The model under review builds one solid part; all positions refer to its coordinate system, in mm. Face numbers are marked on the shaded views. A direction names the side the tool comes from. Coordinates: 2 decimals unless noted, no trailing zeros. Loops run counter-clockwise (first coordinate to the right, second up) from the corner with the lowest first, then second, coordinate; pieces in that order, holes last. Notation, with made-up numbers: (51, 58.25) - (105, 58.25) arc R15 cw to (105, 76.25) - close; hole circle Ø10 at (78.25, -22). An arc over 180 degrees is marked (long way). Answer in a Markdown table with one row per item. Add a question column.
(1) Mouldability with a two-part tool opening along X and no side actions: class the marked faces 1, 2 and 3 as +X half, -X half, draft (parallel to the pull), parting line (faces both ways), or undercut.
(2) We need section D-D on y = -4. Write out the cut boundary in (x, z) (3 decimals).
(3) We need section A-A on z = 0. Write out the cut boundary in (x, y) (3 decimals), plus the area to 3 significant figures.
(4) For P1, Ø8, axis at x = 14, z = -18, coming from the -Y side; P2, Ø8, axis at y = -17, z = 4, coming from the +X side; P3, Ø2, axis at y = -5, z = -3.5, coming from the +X side, all flat-tipped, find the tip position at first contact; note any pin that passes through.
(5) We need section C-C on x = 22.5. Write out the cut boundary in (y, z).
(6) We need section B-B on y = -20. Write out the cut boundary in (x, z).
(7) For line 1 along Y through (x, z) = (16, 1); line 2 along Z through (x, y) = (-1.5, -18); line 3 along X through (y, z) = (-4.5, -18), list the stretches that pass through material, from the lowest coordinate up.
(8) Machinability: for the marked faces 4, 5 and 6, which of the approach directions +Z, -Z, +X, -X, +Y, -Y give a long, thin tool a straight path to every point of the face, cutting with its end or side? Answer none if there is none.
from build123d import *

# Parameters (mm, degrees)
F0_R     = 28.575
F0_R_2   = 2.54
F0_R_3   = 12.192
F1_DEPTH = 6.35
F2_DEPTH = 25.4


with BuildPart() as f1:
    # F0 (on Front) → F1 (new body)
    with BuildSketch(Plane.XZ):
        Circle(F0_R)
        with Locations((-12.7, -20.143117)):
            Circle(F0_R_2, mode=Mode.SUBTRACT)
        with Locations((11.094451, -21.070081)):
            Circle(F0_R_2, mode=Mode.SUBTRACT)
        with Locations((23.794451, -0.926964)):
            Circle(F0_R_2, mode=Mode.SUBTRACT)
        with Locations((-23.794451, 0.926964)):
            Circle(F0_R_2, mode=Mode.SUBTRACT)
        with Locations((-11.094451, 21.070081)):
            Circle(F0_R_2, mode=Mode.SUBTRACT)
        Circle(F0_R_3, mode=Mode.SUBTRACT)
        with Locations((12.7, 20.143117)):
            Circle(F0_R_2, mode=Mode.SUBTRACT)
    extrude(amount=F1_DEPTH)

    # F0 (on Front) → F2 (join)
    with BuildSketch(Plane.XZ):
        Circle(F0_R_3)
        Polygon((-5.500707, 3.186898), (0.009581, 6.357201), (5.510288, 3.170303), (5.500707, -3.186898), (-0.009581, -6.357201), (-5.510288, -3.170303), align=None, mode=Mode.SUBTRACT)
    extrude(amount=F2_DEPTH)


solid = f1.part
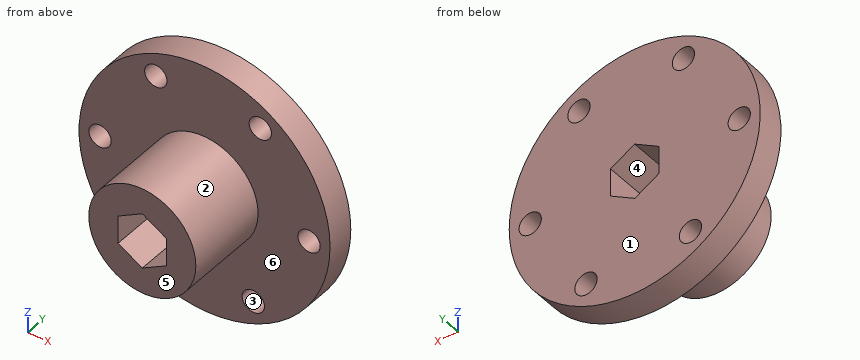
Outcome:
| question | item | result |
|---|---|---|
| 1 | face 1 | draft |
| 1 | face 2 | parting line |
| 1 | face 3 | undercut |
| 2 | outline | circle Ø57.15 at (0, 0); hole circle Ø5.08 at (-23.794, 0.927); hole circle Ø5.08 at (-12.7, -20.143); hole circle Ø5.08 at (-11.094, 21.07); hole (-5.51, -3.17) - (-0.01, -6.357) - (5.501, -3.187) - (5.51, 3.17) - (0.01, 6.357) - (-5.501, 3.187) - close; hole circle Ø5.08 at (11.094, -21.07); hole circle Ø5.08 at (12.7, 20.143); hole circle Ø5.08 at (23.794, -0.927) |
| 3 | outline | (-28.575, -6.35) - (-26.159, -6.35) - (-26.159, 0) - (-28.575, 0) - close; (-21.43, -6.35) - (-12.192, -6.35) - (-12.192, -25.4) - (-5.506, -25.4) - (-5.506, 0) - (-21.43, 0) - close; (5.506, -25.4) - (12.192, -25.4) - (12.192, -6.35) - (21.43, -6.35) - (21.43, 0) - (5.506, 0) - close; (26.159, -6.35) - (28.575, -6.35) - (28.575, 0) - (26.159, 0) - close |
| 3 | area | 488 mm² |
| 4 | P1 | y = -6.35 |
| 4 | P2 | x = 12.19 |
| 4 | P3 | x = 28.47 |
| 5 | outline | (-6.35, -17.61) - (0, -17.61) - (0, -3.11) - (-6.35, -3.11) - close; (-6.35, 1.26) - (0, 1.26) - (0, 17.61) - (-6.35, 17.61) - close |
| 6 | outline | circle Ø24.38 at (0, 0); hole (-5.51, -3.17) - (-0.01, -6.36) - (5.5, -3.19) - (5.51, 3.17) - (0.01, 6.36) - (-5.5, 3.19) - close |
| 7 | line 1 | -6.35 to 0 |
| 7 | line 2 | -12.1 to -5.49, 5.49 to 12.1 |
| 7 | line 3 | -22.19 to -14.06, -11.34 to 22.19 |
| 8 | face 4 | +Y, -Y |
| 8 | face 5 | +Z, -Z, +X, -X, -Y |
| 8 | face 6 | -Y |
